Build history of the part. All positions in model axes, mm. Face numbers are marked on the shaded views. A direction names the side the tool comes from. Give positions to 0.01 mm unless a question says otherwise; leave off trailing zeros. Order: outer loops, then holes, each group sorted by start corner. A loop starts at its lowest first (then second) coordinate and runs counter-clockwise, first axis right, second up. Notation, with made-up numbers: (78, 54.25) - (83, 54.25) arc R15 cw to (83, 71.25) - close; hole circle Ø8 at (71.5, -16.75). An arc over 180 degrees is marked (long way). Use a Markdown table: item, result. Add a question column.
(1) Slice it at A-A (y = 27.5). Write the cut outline in (x, z), then the cut area to 3 significant figures.
(2) Which spindle directions (+Z, -Z, +X, -X, +Y, -Y) get a long thin tool onto all of the face, cutting with end or side? Do the marked faces 5, 6, 7 and 8. Say none if no direction does.
(3) Wall check: line 1 (X direction, y = 18, z = 11); line 2 (X direction, y = 4, z = 7.5); line 3 (Z direction, x = -8, y = 31). Give the ranges that are in metal, low to high.
(4) Flat gauge pins, fed straight in: pin 1 (5 mm diameter, centred on x = -2, z = 15, fed in from -Y); pin 2 (8 mm diameter, centred on x = 1.5, z = -4.5, fed in from +Y); pin 3 (6.5 mm diameter, centred on x = 6.5, y = 17.5, fed in from -Z). Where does each tip first touch, or does it go through?
(5) Mould opens along Y. For the marked faces 1, 2, 3 and 4 say: +Y half, -Y half, draft (parallel to the pull), parting line (faces both ways), or undercut.
(6) Slice it at D-D (z = 8). Write the cut outline in (x, y).
(7) Slice it at B-B (x = 1.25). Write the cut outline in (y, z), then the cut area to 3 significant figures.
(8) Slice it at C-C (z = -5.75). Write the cut outline in (x, y), then the cut area to 3 significant figures.
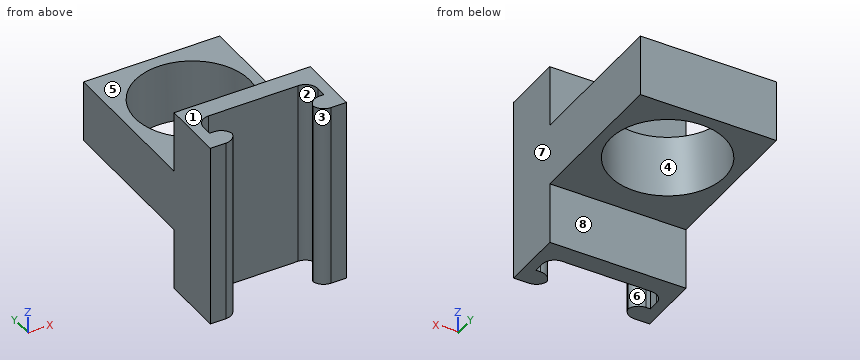
from build123d import *

# Parameters (mm, degrees)
SKETCH1_W           = 22
SKETCH1_H           = 30
BOSS_EXTRUDE1_DEPTH = 10
CUT_EXTRUDE1_DEPTH  = 34.925879042
FILLET1_R           = 2
SKETCH4_W           = 22
SKETCH4_H           = 10
BOSS_EXTRUDE2_DEPTH = 25
CUT_EXTRUDE2_REACH  = 44.142
SKETCH5_R           = 9.25


with BuildPart() as part:
    # Sketch1 → Boss-Extrude1 (new body)
    with BuildSketch(Plane(origin=(0, 0, 0), x_dir=(1, 0, 0), z_dir=(0, 1, 0))):
        with Locations((1.286792453, -6.677358491)):
            Rectangle(SKETCH1_W, SKETCH1_H)
    extrude(amount=BOSS_EXTRUDE1_DEPTH)

    # Sketch2 → Cut-Extrude1 (cut, through all)
    with BuildSketch(Plane.XY.offset(21.677358491)):
        Polygon((-7.963207547, 6.9), (10.536792453, 6.9), (10.536792453, 3.2), (7.786792453, 3.2), (7.786792453, 0), (-5.213207547, 0), (-5.213207547, 3.2), (-7.963207547, 3.2), align=None)
    extrude(amount=-CUT_EXTRUDE1_DEPTH, mode=Mode.SUBTRACT)

    # Fillet1
    # the kernel refuses this fillet: 2 mm, written as the material it adds along each edge
    with BuildSketch(Plane(origin=(10.536792453, 6.9, 21.677358491), x_dir=(-1, 0, 0), z_dir=(0, 0, -1)), Plane(origin=(-7.963207547, 6.9, 21.677358491), x_dir=(0, -1, 0), z_dir=(0, 0, -1))) as fillet1_piece_1:
        with BuildLine():
            CenterArc((FILLET1_R, -FILLET1_R), FILLET1_R, 90, 90)
            Line((0, -FILLET1_R), (0, 0))
            Line((0, 0), (FILLET1_R, 0))
        make_face()
    extrude(amount=30)
    # the kernel refuses this fillet: 2 mm, written as the material it takes off along each edge
    with BuildSketch(Plane(origin=(-5.213207547, 0, 26.677358491), x_dir=(-1, 0, 0), z_dir=(0, 0, -1)), Plane(origin=(7.786792453, 0, 26.677358491), x_dir=(0, 1, 0), z_dir=(0, 0, -1)), Plane(origin=(7.786792453, 3.2, 26.677358491), x_dir=(1, 0, 0), z_dir=(0, 0, -1)), Plane(origin=(-5.213207547, 3.2, 26.677358491), x_dir=(0, -1, 0), z_dir=(0, 0, -1))) as fillet1_2_piece_1:
        with BuildLine():
            CenterArc((FILLET1_R, FILLET1_R), FILLET1_R, 180, 90)
            Line((0, FILLET1_R), (0, 0))
            Line((0, 0), (FILLET1_R, 0))
        make_face()
    extrude(amount=40, mode=Mode.SUBTRACT)

    # Sketch4 → Boss-Extrude2 (add)
    with BuildSketch(Plane(origin=(0, 10, 0), x_dir=(1, 0, 0), z_dir=(0, 1, 0))):
        with Locations((1.286792453, -6.677358491)):
            Rectangle(SKETCH4_W, SKETCH4_H)
    extrude(amount=BOSS_EXTRUDE2_DEPTH)

    # Sketch5 → Cut-Extrude2 (cut, up to next)
    with BuildSketch(Plane.XY.offset(11.677358491), mode=Mode.PRIVATE) as cut_extrude2_sk1:
        with Locations((1.286792453, 23.746)):
            Circle(SKETCH5_R)
    cut_extrude2_tool1 = extrude(cut_extrude2_sk1.sketch, amount=-CUT_EXTRUDE2_REACH, mode=Mode.PRIVATE) & part.part
    add(cut_extrude2_tool1.solids().sort_by_distance((1.286792, 23.746, 11.677358))[0], mode=Mode.SUBTRACT)


solid = part.part
Solution:
| question | item | result |
|---|---|---|
| 1 | outline | (-9.71, 1.68) - (-7.17, 1.68) - (-7.17, 11.68) - (-9.71, 11.68) - close; (9.74, 1.68) - (12.29, 1.68) - (12.29, 11.68) - (9.74, 11.68) - close |
| 1 | area | 50.9 mm2 |
| 2 | face 5 | +Z, +X, -X, +Y |
| 2 | face 6 | +Z, -Z |
| 2 | face 7 | +Z, -Z, +X, +Y, -Y |
| 2 | face 8 | -Z, +X, -X, +Y |
| 3 | line 1 | -9.71 to -5.96, 8.54 to 12.29 |
| 3 | line 2 | -9.71 to -7.96, 10.54 to 12.29 |
| 3 | line 3 | 1.68 to 11.68 |
| 4 | pin 1 | y = 6.9 |
| 4 | pin 2 | y = 10 |
| 4 | pin 3 | z = 1.68 |
| 5 | face 1 | draft |
| 5 | face 2 | undercut |
| 5 | face 3 | -Y half |
| 5 | face 4 | undercut |
| 6 | outline | (-9.71, 0) - (-7.21, 0) arc R2 ccw to (-5.25, 1.6) arc R2 ccw to (-7.21, 3.2) - (-7.96, 3.2) - (-7.96, 4.9) arc R2 cw to (-5.96, 6.9) - (8.54, 6.9) arc R2 cw to (10.54, 4.9) - (10.54, 3.2) - (9.79, 3.2) arc R2 ccw to (7.83, 1.6) arc R2 ccw to (9.79, 0) - (12.29, 0) - (12.29, 35) - (-9.71, 35) - close; hole circle Ø18.5 at (1.29, 23.75) |
| 7 | outline | (6.9, -8.32) - (10, -8.32) - (10, 1.68) - (14.5, 1.68) - (14.5, 11.68) - (10, 11.68) - (10, 21.68) - (6.9, 21.68) - close; (33, 1.68) - (35, 1.68) - (35, 11.68) - (33, 11.68) - close |
| 7 | area | 158 mm2 |
| 8 | outline | (-9.71, 0) - (-7.21, 0) arc R2 ccw to (-5.25, 1.6) arc R2 ccw to (-7.21, 3.2) - (-7.96, 3.2) - (-7.96, 4.9) arc R2 cw to (-5.96, 6.9) - (8.54, 6.9) arc R2 cw to (10.54, 4.9) - (10.54, 3.2) - (9.79, 3.2) arc R2 ccw to (7.83, 1.6) arc R2 ccw to (9.79, 0) - (12.29, 0) - (12.29, 10) - (-9.71, 10) - close |
| 8 | area | 108 mm2 |
